For this review, take the finished solid that the model builds, in its own axes (mm). Coordinates: 2 decimals unless noted, no trailing zeros. Write each loop counter-clockwise with the first axis right and the second up, starting at its lowest first coordinate (ties: lowest second). Pieces come first, ordered by that corner, then holes. Notation, with made-up numbers: (-15, 20) -> (11, 20) arc R23 cw to (11, 55) -> close; hole circle Ø8 at (49, -30). An arc over 180 degrees is marked (long way). One line per item, written item: value. Start each with the question number.
1) Add section D-D (x = 61.5). State the section outline as (y, z) points.
2) For probe 1 along Z at (x, y) = (64, 16); probe 2 along Y at (x, z) = (10, -26.7); probe 3 along Y at (x, z) = (45, -27.1), list the stretches that pass through material, from the lowest coordinate up. Write a range as from..to.
3) Add section B-B (y = 15). State the section outline as (x, z) points.
4) Add section A-A (x = 38). State the section outline as (y, z) points.
5) Mouldability with a two-part tool opening along Z and no side actions: class faces 1 (the cylindrical face through (43.5, 0.99, -21.07)), 2 (the cylindrical face through (42.05, 0.99, -16.7)), 3 (the cylindrical face through (1.5, 40.43, -0.99)) as released by +Z, released by -Z, zero draft, split by the parting line, or undercut.
6) For pin 1 Ø2.5 at (x, y) = (10, 22.86) entering from +Z; pin 2 Ø3.5 at (x, y) = (10, 22.86) entering from -Z; pin 3 Ø8 at (x, z) = (69.5, -15) entering from +Y, all flat-tipped, find the tip position at first contact; note any pin that passes through.
7) Add section C-C (z = -14). State how many separate pieces and enclosed holes the cut face has, and give its area (3 significant figures).
from build123d import *

# Parameters (mm, degrees)
ESTRUSIONE_ESTRUSIONE1_DEPTH = 2
SCHIZZO2_W                   = 90
SCHIZZO2_H                   = 28
ESTRUSIONE_ESTRUSIONE2_DEPTH = 2
ESTRUSIONE_ESTRUSIONE3_DEPTH = 2
SCHIZZO5_R                   = 4
SCHIZZO5_R_2                 = 1.5
TAGLIO_ESTRUSIONE1_DEPTH     = 29
RACCORDO1_R                  = 2
RACCORDO2_R                  = 2
RACCORDO3_R                  = 1
RACCORDO4_R                  = 1
SCHIZZO6_R                   = 4
SCHIZZO6_R_2                 = 1.5
TAGLIO_ESTRUSIONE2_DEPTH     = 42.860465116
SKETCH1_R                    = 1.5
CUT_EXTRUDE1_DEPTH           = 1
CUT_EXTRUDE1_DEPTH_BACK      = 29


with BuildPart() as part:
    # Schizzo1 → Estrusione-Estrusione1 (new body)
    with BuildSketch(Plane.XY):
        with BuildLine():
            Line((0, 0), (90, 0))
            Line((90, 0), (90, 36.860465116))
            ThreePointArc((90, 36.860465116), (88.535533906, 40.395999022), (85, 41.860465116))
            Line((85, 41.860465116), (5, 41.860465116))
            ThreePointArc((5, 41.860465116), (1.464466094, 40.395999022), (0, 36.860465116))
            Line((0, 36.860465116), (0, 0))
        make_face()
    extrude(amount=-ESTRUSIONE_ESTRUSIONE1_DEPTH)

    # Schizzo2 → Estrusione-Estrusione2 (add)
    with BuildSketch(Plane(origin=(0, 0, 0), x_dir=(1, 0, 0), z_dir=(0, 1, 0))):
        with Locations((45, 14)):
            Rectangle(SCHIZZO2_W, SCHIZZO2_H)
    extrude(amount=ESTRUSIONE_ESTRUSIONE2_DEPTH)

    # Schizzo4 → Estrusione-Estrusione3 (add)
    with BuildSketch(Plane.XY.offset(-28)):
        with BuildLine():
            Line((90, 0), (90, 36.860465116))
            ThreePointArc((90, 36.860465116), (88.535533906, 40.395999022), (85, 41.860465116))
            Line((85, 41.860465116), (5, 41.860465116))
            ThreePointArc((5, 41.860465116), (1.464466094, 40.395999022), (0, 36.860465116))
            Line((0, 36.860465116), (0, 0))
            Line((0, 0), (90, 0))
        make_face()
    extrude(amount=ESTRUSIONE_ESTRUSIONE3_DEPTH)

    # Schizzo5 → Taglio-Estrusione1 (cut, through all)
    with BuildSketch(Plane.XY):
        with Locations((10, 29.860465116)):
            Circle(SCHIZZO5_R)
        with Locations((45, 29.860465116)):
            Circle(SCHIZZO5_R)
        with Locations((80, 29.860465116)):
            Circle(SCHIZZO5_R)
        with Locations((10, 36.860465116)):
            Circle(SCHIZZO5_R_2)
        with Locations((3, 29.860465116)):
            Circle(SCHIZZO5_R_2)
        with Locations((10, 22.860465116)):
            Circle(SCHIZZO5_R_2)
        with Locations((17, 29.860465116)):
            Circle(SCHIZZO5_R_2)
        with Locations((38, 29.860465116)):
            Circle(SCHIZZO5_R_2)
        with Locations((45, 36.860465116)):
            Circle(SCHIZZO5_R_2)
        with Locations((80, 36.860465116)):
            Circle(SCHIZZO5_R_2)
        with Locations((73, 29.860465116)):
            Circle(SCHIZZO5_R_2)
        with Locations((45, 22.860465116)):
            Circle(SCHIZZO5_R_2)
        with Locations((80, 22.860465116)):
            Circle(SCHIZZO5_R_2)
        with Locations((87, 29.860465116)):
            Circle(SCHIZZO5_R_2)
        with Locations((52, 29.860465116)):
            Circle(SCHIZZO5_R_2)
    extrude(amount=-TAGLIO_ESTRUSIONE1_DEPTH, mode=Mode.SUBTRACT)

    # Raccordo1
    raccordo1_edges = [part.edges().sort_by_distance(p)[0] for p in [
        (45, 0, -28),
    ]]
    fillet(raccordo1_edges, radius=RACCORDO1_R)

    # Raccordo2
    raccordo2_edges = [part.edges().sort_by_distance(p)[0] for p in [
        (45, 0, 0),
    ]]
    fillet(raccordo2_edges, radius=RACCORDO2_R)

    # Raccordo3
    raccordo3_edges = [part.edges().sort_by_distance(p)[0] for p in [
        (45, 2, -2),
    ]]
    fillet(raccordo3_edges, radius=RACCORDO3_R)

    # Raccordo4
    raccordo4_edges = [part.edges().sort_by_distance(p)[0] for p in [
        (45, 2, -26),
    ]]
    fillet(raccordo4_edges, radius=RACCORDO4_R)

    # Schizzo6 → Taglio-Estrusione2 (cut, through all)
    with BuildSketch(Plane(origin=(0, 0, 0), x_dir=(1, 0, 0), z_dir=(0, 1, 0))):
        with Locations((45, 14)):
            Circle(SCHIZZO6_R)
        with Locations((10, 14)):
            Circle(SCHIZZO6_R)
        with Locations((80, 14)):
            Circle(SCHIZZO6_R)
        with Locations((10, 21)):
            Circle(SCHIZZO6_R_2)
        with Locations((3, 14)):
            Circle(SCHIZZO6_R_2)
        with Locations((10, 7)):
            Circle(SCHIZZO6_R_2)
        with Locations((17, 14)):
            Circle(SCHIZZO6_R_2)
        with Locations((38, 14)):
            Circle(SCHIZZO6_R_2)
        with Locations((45, 21)):
            Circle(SCHIZZO6_R_2)
        with Locations((80, 21)):
            Circle(SCHIZZO6_R_2)
        with Locations((80, 7)):
            Circle(SCHIZZO6_R_2)
        with Locations((45, 7)):
            Circle(SCHIZZO6_R_2)
        with Locations((52, 14)):
            Circle(SCHIZZO6_R_2)
        with Locations((87, 14)):
            Circle(SCHIZZO6_R_2)
        with Locations((73, 14)):
            Circle(SCHIZZO6_R_2)
    extrude(amount=TAGLIO_ESTRUSIONE2_DEPTH, mode=Mode.SUBTRACT)

    # Sketch1 → Cut-Extrude1 (cut, two sides)
    with BuildSketch(Plane.XY) as cut_extrude1_sk:
        with Locations((31.5, 36.860465116)):
            Circle(SKETCH1_R)
        with Locations((58.5, 36.860465116)):
            Circle(SKETCH1_R)
    extrude(amount=CUT_EXTRUDE1_DEPTH, mode=Mode.SUBTRACT)
    extrude(cut_extrude1_sk.sketch, amount=-CUT_EXTRUDE1_DEPTH_BACK, mode=Mode.SUBTRACT)


solid = part.part
Numbers:
1. outline: (0, -26) arc R2 ccw to (2, -28) -> (41.86, -28) -> (41.86, -26) -> (3, -26) arc R1 cw to (2, -25) -> (2, -3) arc R1 cw to (3, -2) -> (41.86, -2) -> (41.86, 0) -> (2, 0) arc R2 ccw to (0, -2) -> close
2. probe 1: -28..-26, -2..0
2. probe 2: 0.13..21.36, 24.36..25.86, 33.86..35.36, 38.36..41.86
2. probe 3: 0.33..21.36, 24.36..25.86, 33.86..35.36, 38.36..41.86
3. outline: (0, -28) -> (90, -28) -> (90, -26) -> (0, -26) -> close; (0, -2) -> (90, -2) -> (90, 0) -> (0, 0) -> close
4. outline: (0, -26) arc R2 ccw to (2, -28) -> (28.36, -28) -> (28.36, -26) -> (3, -26) arc R1 cw to (2, -25) -> (2, -15.5) -> (0, -15.5) -> close; (0, -12.5) -> (2, -12.5) -> (2, -3) arc R1 cw to (3, -2) -> (28.36, -2) -> (28.36, 0) -> (2, 0) arc R2 ccw to (0, -2) -> close; (31.36, -28) -> (41.86, -28) -> (41.86, -26) -> (31.36, -26) -> close; (31.36, -2) -> (41.86, -2) -> (41.86, 0) -> (31.36, 0) -> close
5. face 1: undercut
5. face 2: undercut
5. face 3: zero draft
6. pin 1: through
6. pin 2: z = -28
6. pin 3: y = 2
7. separate pieces: 10
7. enclosed holes: 0
7. area: 96.0 mm²
